from build123d import *

# Parameters (mm, degrees)
SKETCH1_W                   = 107
SKETCH1_H                   = 60
BOSS_EXTRUDE1_DEPTH         = 5
SKETCH2_W                   = 60
SKETCH2_H                   = 17
CUT_EXTRUDE1_DEPTH          = 2
CHAMFER1_SIZE               = 2
CHAMFER2_SIZE               = 3
FILLET1_R                   = 1
TAP_DRILL_FOR_M5_TAP1_D     = 4.2
TAP_DRILL_FOR_M5_TAP1_DEPTH = 46
TAP_DRILL_FOR_M5_TAP1_TIP   = 1.2618073
TAP_DRILL_FOR_M5_TAP2_D     = 4.2
TAP_DRILL_FOR_M5_TAP2_DEPTH = 46
TAP_DRILL_FOR_M5_TAP2_TIP   = 1.2618073


with BuildPart() as part:
    # Sketch1 → Boss-Extrude1 (new body)
    with BuildSketch(Plane(origin=(0, 0, 0), x_dir=(1, 0, 0), z_dir=(0, 1, 0))):
        Rectangle(SKETCH1_W, SKETCH1_H)
    extrude(amount=BOSS_EXTRUDE1_DEPTH)

    # Sketch2 → Cut-Extrude1 (cut)
    with BuildSketch(Plane(origin=(0, 5, 0), x_dir=(1, 0, 0), z_dir=(0, 1, 0))):
        with Locations((0, -21.5)):
            Rectangle(SKETCH2_W, SKETCH2_H)
    extrude(amount=-CUT_EXTRUDE1_DEPTH, mode=Mode.SUBTRACT)

    # Chamfer1
    chamfer1_edges = [part.edges().sort_by_distance(p)[0] for p in [
        (30, 4, 13),
        (30, 4, 30),
        (-30, 4, 30),
        (-30, 4, 13),
    ]]
    chamfer(chamfer1_edges, length=CHAMFER1_SIZE)

    # Chamfer2
    chamfer2_edges = [part.edges().sort_by_distance(p)[0] for p in [
        (53.5, 2.5, 30),
        (-53.5, 2.5, 30),
        (-53.5, 2.5, -30),
        (53.5, 2.5, -30),
    ]]
    chamfer(chamfer2_edges, length=CHAMFER2_SIZE)

    # Fillet1
    fillet1_edges = [part.edges().sort_by_distance(p)[0] for p in [
        (30, 4, 15),
        (30, 4, 28),
        (-32, 4, 30),
        (32, 4, 30),
        (-28, 4, 13),
        (28, 4, 13),
        (-30, 4, 15),
        (-30, 4, 28),
        (-53.5, 2.5, 27),
        (-53.5, 2.5, -27),
        (50.5, 2.5, -30),
        (-50.5, 2.5, -30),
        (50.5, 2.5, 30),
        (-50.5, 2.5, 30),
        (53.5, 2.5, 27),
        (53.5, 2.5, -27),
    ]]
    fillet(fillet1_edges, radius=FILLET1_R)

    # Tap Drill for M5 Tap1
    with Locations(Plane(origin=(-41.25, 5, 21), x_dir=(0, 0, 1), z_dir=(0, 1, 0))):
        with Locations((0, 0), (-41, 0), (-41, 41.25), (-41, 82.5), (0, 82.5)):
            Hole(TAP_DRILL_FOR_M5_TAP1_D / 2, depth=TAP_DRILL_FOR_M5_TAP1_DEPTH)
            with Locations((0, 0, -(TAP_DRILL_FOR_M5_TAP1_DEPTH + TAP_DRILL_FOR_M5_TAP1_TIP / 2))):  # 118° drill point
                Cone(0, TAP_DRILL_FOR_M5_TAP1_D / 2, TAP_DRILL_FOR_M5_TAP1_TIP, mode=Mode.SUBTRACT)

    # Tap Drill for M5 Tap2
    with Locations(Plane(origin=(-19, 3, 21), x_dir=(0, 0, 1), z_dir=(0, 1, 0))):
        with Locations((0, 0), (0, 38)):
            Hole(TAP_DRILL_FOR_M5_TAP2_D / 2, depth=TAP_DRILL_FOR_M5_TAP2_DEPTH)
            with Locations((0, 0, -(TAP_DRILL_FOR_M5_TAP2_DEPTH + TAP_DRILL_FOR_M5_TAP2_TIP / 2))):  # 118° drill point
                Cone(0, TAP_DRILL_FOR_M5_TAP2_D / 2, TAP_DRILL_FOR_M5_TAP2_TIP, mode=Mode.SUBTRACT)


solid = part.part
Input: part model. Units: mm. Frame: model coordinates. A direction names the side the tool comes from. Coordinates: 2 decimals unless noted, no trailing zeros. Loops run counter-clockwise (first coordinate to the right, second up) from the corner with the lowest first, then second, coordinate; pieces in that order, holes last. Notation, with made-up numbers: (3.5, 74) -> (25.5, 74) arc R19 ccw to (25.5, 87) -> close; hole circle Ø1 at (-5, -9). An arc over 180 degrees is marked (long way). Write item = value, one per line. Start each with the question number.
Item 1: Mould query, pull axis Z, two halves, no side actions, for faces 3 (the face through (52, 2.5, 28.5)), 4 (the face through (52, 2.5, -28.5)), 5 (the face through (39.387, 2.465, 20.031)). Classes: pulls with the +Z half, pulls with the -Z half, needs draft (parallel to the pull), parting line crosses it, or undercut.
Item 2: Material intervals for line 1 (X direction, y = 3.9, z = -20); line 2 (X direction, y = 1.5, z = 21); line 3 (X direction, y = 4.6, z = -21), sorted ascending.
Item 3: First-contact query: P1, Ø4, axis at x = -41.25, z = 21, coming from the +Y side; P2, Ø6.5, axis at x = 19, z = 21, coming from the +Y side. Flat tips, straight axial feed; report the tip coordinate or a pass-through.
Item 4: Cut plane B-B, the plane z = -20. Return loops of the section in (x, y).
Item 5: Cut plane A-A, the plane x = 19. Return loops of the section in (y, z).
Item 6: Cut plane D-D, the plane z = 21. Return loops of the section in (x, y).
Item 7: Cut plane C-C, the plane y = 1.35. Return loops of the section in (x, z).
Item 8: Reachability of faces 1 (the face through (-43.113, 2.465, -20.969)), 2 (the face through (-30, 4, 22)) from +Z, -Z, +X, -X, +Y, -Y: full face, straight path, thin tool, end or side. Return the list, or none.
Ans:
q1.face_3 = pulls with the +Z half
q1.face_4 = pulls with the -Z half
q1.face_5 = undercut
q2.line_1 = -53.5 to -43.35, -39.15 to -2.1, 2.1 to 39.15, 43.35 to 53.5
q2.line_2 = -53.5 to -43.35, -39.15 to -21.1, -16.9 to 16.9, 21.1 to 39.15, 43.35 to 53.5
q2.line_3 = -53.5 to -43.1, -39.4 to -1.85, 1.85 to 39.4, 43.1 to 53.5
q3.P1 = through
q3.P2 = 3
q4.outline = (-53.5, 0) -> (-43.35, 0) -> (-43.35, 5) -> (-53.5, 5) -> close; (-39.15, 0) -> (-2.1, 0) -> (-2.1, 5) -> (-39.15, 5) -> close; (2.1, 0) -> (39.15, 0) -> (39.15, 5) -> (2.1, 5) -> close; (43.35, 0) -> (53.5, 0) -> (53.5, 5) -> (43.35, 5) -> close
q5.outline = (0, -30) -> (5, -30) -> (5, 13) -> (3, 13) -> (3, 18.9) -> (0, 18.9) -> close; (0, 23.1) -> (3, 23.1) -> (3, 30) -> (0, 30) -> close
q6.outline = (-53.5, 0) -> (-43.35, 0) -> (-43.35, 5) -> (-53.5, 5) -> close; (-39.15, 0) -> (-21.1, 0) -> (-21.1, 3) -> (-30, 3) -> (-30, 5) -> (-39.15, 5) -> close; (-16.9, 0) -> (16.9, 0) -> (16.9, 3) -> (-16.9, 3) -> close; (21.1, 0) -> (39.15, 0) -> (39.15, 5) -> (30, 5) -> (30, 3) -> (21.1, 3) -> close; (43.35, 0) -> (53.5, 0) -> (53.5, 5) -> (43.35, 5) -> close
q7.outline = (-53.5, -26.59) arc R1 ccw to (-53.21, -27.29) -> (-50.79, -29.71) arc R1 ccw to (-50.09, -30) -> (50.09, -30) arc R1 ccw to (50.79, -29.71) -> (53.21, -27.29) arc R1 ccw to (53.5, -26.59) -> (53.5, 26.59) arc R1 ccw to (53.21, 27.29) -> (50.79, 29.71) arc R1 ccw to (50.09, 30) -> (-50.09, 30) arc R1 ccw to (-50.79, 29.71) -> (-53.21, 27.29) arc R1 ccw to (-53.5, 26.59) -> close; hole circle Ø4.2 at (-41.25, -20); hole circle Ø4.2 at (-41.25, 21); hole circle Ø4.2 at (-19, 21); hole circle Ø4.2 at (0, -20); hole circle Ø4.2 at (19, 21); hole circle Ø4.2 at (41.25, -20); hole circle Ø4.2 at (41.25, 21)
q8.face_1 = +Y, -Y
q8.face_2 = +Z, +Y
